from build123d import *

# Parameters (mm, degrees)
F0_W      = 50.8
F0_H      = 50.8
F1_DEPTH  = 12.7
F2_W      = 9.9903053224
F2_H      = 20.6871938426
F3_DEPTH  = 25.4
F4_R      = 2.54
F5_DEPTH  = 25.4
F6_R      = 2.54
F7_DEPTH  = 7.874
F8_R      = 2.54
F9_DEPTH  = 12.7
F10_R     = 2.54
F11_DEPTH = 7.62


with BuildPart() as f1:
    # F0 (on Top) → F1 (new body)
    with BuildSketch(Plane.XY):
        Rectangle(F0_W, F0_H)
    extrude(amount=F1_DEPTH)

    # F2 (on face) → F3 (cut)
    with BuildSketch(Plane.XY.offset(12.7)):
        with Locations((20.4048473388, 0.4619845422)):
            Rectangle(F2_W, F2_H)
    extrude(amount=-F3_DEPTH, mode=Mode.SUBTRACT)

    # F4 (on face) → F5 (cut)
    with BuildSketch(Plane.XY.offset(12.7)):
        with Locations((-15, 15)):
            Circle(F4_R)
        with Locations((15, 15)):
            Circle(F4_R)
        with Locations((-15, -15)):
            Circle(F4_R)
        with Locations((15, -15)):
            Circle(F4_R)
    extrude(amount=-F5_DEPTH, mode=Mode.SUBTRACT)

    # F6 (on face) → F7 (cut)
    with BuildSketch(Plane.XZ.offset(25.4)):
        with Locations((0, 7.62)):
            Circle(F6_R)
    extrude(amount=-F7_DEPTH, mode=Mode.SUBTRACT)

    # F8 (on face) → F9 (cut)
    with BuildSketch(Plane(origin=(-25.4, 0, 0), x_dir=(0, -1, 0), z_dir=(-1, 0, 0))):
        with Locations((0, 7.62)):
            Circle(F8_R)
    extrude(amount=-F9_DEPTH, mode=Mode.SUBTRACT)

    # F10 (on face) → F11 (cut)
    with BuildSketch(Plane(origin=(0, 25.4, 0), x_dir=(-1, 0, 0), z_dir=(0, 1, 0))):
        with Locations((0, 7.62)):
            Circle(F10_R)
    extrude(amount=-F11_DEPTH, mode=Mode.SUBTRACT)


solid = f1.part
Read the model definition and answer for the solid it produces. Units are mm, in the model's axes. A direction names the side the tool comes from. Round coordinates to 2 decimals unless told otherwise and drop trailing zeros. Write each loop counter-clockwise with the first axis right and the second up, starting at its lowest first coordinate (ties: lowest second). Pieces come first, ordered by that corner, then holes.
Q1. Find section B-B on y = 15. Determine the outline of the cut face in (x, z), and give its area (3 significant figures).
Values:
outline: (-25.4, 0) - (-17.54, 0) - (-17.54, 12.7) - (-25.4, 12.7) - close; (-12.46, 0) - (12.46, 0) - (12.46, 12.7) - (-12.46, 12.7) - close; (17.54, 0) - (25.4, 0) - (25.4, 12.7) - (17.54, 12.7) - close
area: 516 mm2
Q2. The mould has two halves that part along Z. Classify faces 1 (the face through (0, 0, 0)), 2 (the face through (-19.14, 0.55, 5.14)), 3 (the face through (25.4, 18, 6)): released by +Z, released by -Z, zero draft, split by the parting line, or undercut.
Values:
face 1: released by -Z
face 2: undercut
face 3: zero draft
Q3. Find section C-C on z = 2.5. Determine the outline of the cut face in (x, y).
Values:
outline: (-25.4, -25.4) - (25.4, -25.4) - (25.4, -9.88) - (15.41, -9.88) - (15.41, 10.81) - (25.4, 10.81) - (25.4, 25.4) - (-25.4, 25.4) - close; hole circle Ø5.08 at (-15, -15); hole circle Ø5.08 at (-15, 15); hole circle Ø5.08 at (15, -15); hole circle Ø5.08 at (15, 15)
Q4. A tool of negligible diameter and unlimited length cuts with its end or side. For faces 4 (the face through (-12.7, 0, 8)), 5 (the face through (20, 10.806, 6)), 6 (the face through (-0.55, -21.52, 5.14)), from which of +Z, -Z, +X, -X, +Y, -Y can it reach the whole face along a straight path? Write none if from no direction.
Values:
face 4: -X
face 5: +Z, -Z, +X
face 6: -Y
Q5. Find section A-A on x = -15. Determine the outline of the cut face in (y, z).
Values:
outline: (-25.4, 0) - (-17.54, 0) - (-17.54, 12.7) - (-25.4, 12.7) - close; (-12.46, 0) - (12.46, 0) - (12.46, 12.7) - (-12.46, 12.7) - close; (17.54, 0) - (25.4, 0) - (25.4, 12.7) - (17.54, 12.7) - close; hole circle Ø5.08 at (0, 7.62)
Q6. Straight lines are drawn through the part: line 1 (Y direction, x = 15, z = 5.75); line 2 (Y direction, x = -16.5, z = 9.25); line 3 (Y direction, x = 22, z = 4). For each, find the intervals that lie inside material, in ascending order.
Values:
line 1: y = -25.4 to -17.54, -12.46 to 12.46, 17.54 to 25.4
line 2: y = -25.4 to -17.05, -12.95 to -1.95, 1.95 to 12.95, 17.05 to 25.4
line 3: y = -25.4 to -9.88, 10.81 to 25.4
Q7. Flat-ended cylindrical pins translate along their axes: P1, Ø3, axis at y = 3, z = 10, coming from the +X side; P2, Ø4.5, axis at x = 0, z = 7.62, coming from the -Y side; P3, Ø4.5, axis at x = 0, z = 7.62, coming from the +Y side; P4, Ø4.5, axis at x = -15, y = 15, coming from the -Z side. Find the tip coordinate at first contact, or state that the pin passes through.
Values:
P1: stops at x = 15.41
P2: stops at y = -17.53
P3: stops at y = 17.78
P4: passes through
Q8. Find section D-D on x = 0. Determine the outline of the cut face in (y, z), and give its area (3 significant figures).
Values:
outline: (-25.4, 0) - (25.4, 0) - (25.4, 5.08) - (17.78, 5.08) - (17.78, 10.16) - (25.4, 10.16) - (25.4, 12.7) - (-25.4, 12.7) - (-25.4, 10.16) - (-17.53, 10.16) - (-17.53, 5.08) - (-25.4, 5.08) - close
area: 566 mm2
